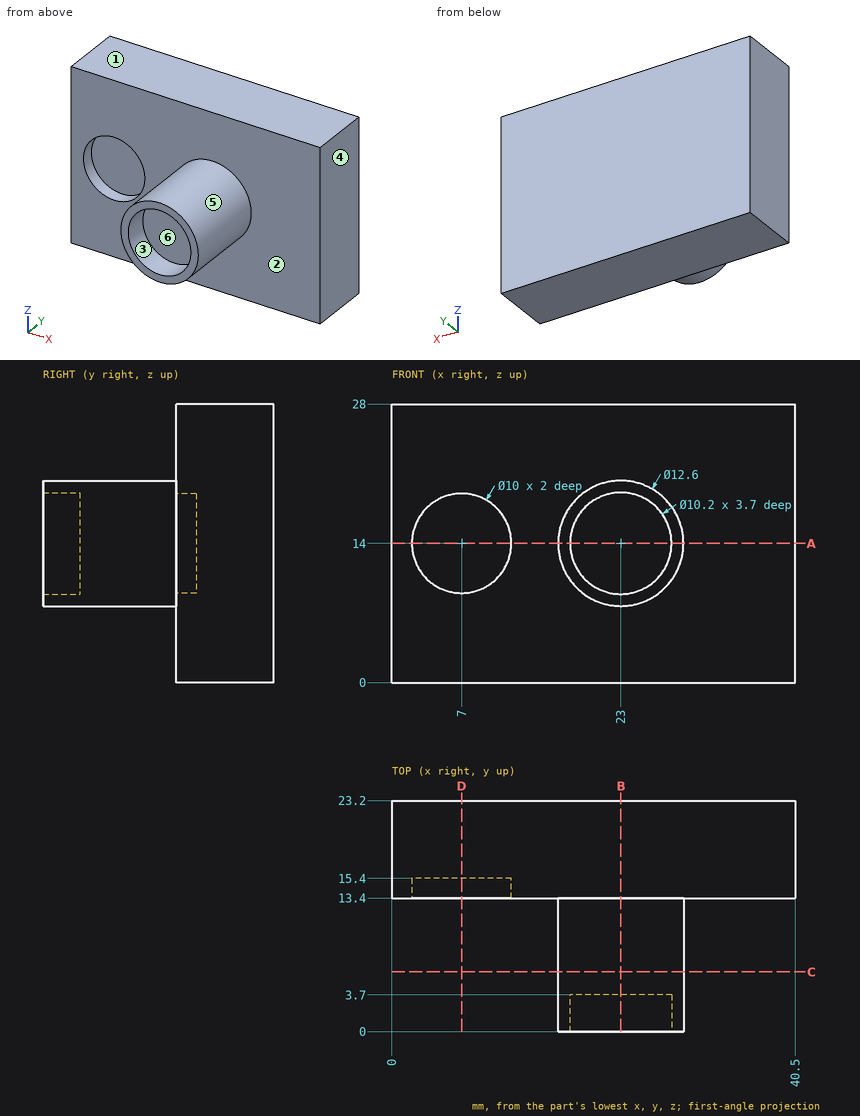
The figure shows three views and two pictorial views of one solid part (mm, origin at its lowest corner). Answer the questions. A direction names the side the tool comes from. Give positions to 0.01 mm unless a question says otherwise; leave off trailing zeros. Write each loop counter-clockwise with the first axis right and the second up, starting at its lowest first coordinate (ties: lowest second). Pieces come first, ordered by that corner, then holes. Notation, with made-up numbers: (-26, 11.5) -> (33, 11.5) arc R25 cw to (33, 38.5) -> close; hole circle Ø6 at (-27.75, 51.5). An arc over 180 degrees is marked (long way). Answer as a JSON object with one key per item and string values.
1) Straight lines are drawn through the part: probe 1 along Z at (x, y) = (7, 13.9); probe 2 along Z at (x, y) = (23, 2.1); probe 3 along Y at (x, z) = (34.5, 16.25). For each, find the intervals that lie inside material, in ascending order. Write a range as from..to.
Findings below:
{"probe 1": "z = 0..9, 19..28", "probe 2": "z = 7.7..8.9, 19.1..20.3", "probe 3": "y = 13.4..23.2"}
2) Flat-ended cylindrical pins translate along their axes: pin 1 Ø5 at (x, z) = (21, 12.5) entering from -Y; pin 2 Ø12 at (y, z) = (12, 23.5) entering from -X; pin 3 Ø8 at (y, z) = (5, 6) entering from -X; pin 4 Ø8 at (x, z) = (7, 14) entering from -Y. Find the tip coordinate at first contact, or state that the pin passes through.
Findings below:
{"pin 1": "stops at y = 3.7", "pin 2": "stops at x = 0", "pin 3": "stops at x = 18.13", "pin 4": "stops at y = 15.4"}
3) Section A-A on z = 14 is taken. Write down the section's boundary in (x, y), then the cut area to 3 significant figures.
Findings below:
{"outline": "(0, 13.4) -> (2, 13.4) -> (2, 15.4) -> (12, 15.4) -> (12, 13.4) -> (16.7, 13.4) -> (16.7, 0) -> (17.9, 0) -> (17.9, 3.7) -> (28.1, 3.7) -> (28.1, 0) -> (29.3, 0) -> (29.3, 13.4) -> (40.5, 13.4) -> (40.5, 23.2) -> (0, 23.2) -> close", "area": "508 mm^2"}
4) Section B-B on x = 23 is taken. Write down the section's boundary in (y, z).
Findings below:
{"outline": "(0, 7.7) -> (13.4, 7.7) -> (13.4, 0) -> (23.2, 0) -> (23.2, 28) -> (13.4, 28) -> (13.4, 20.3) -> (0, 20.3) -> (0, 19.1) -> (3.7, 19.1) -> (3.7, 8.9) -> (0, 8.9) -> close"}
5) For a pull along X with two mould halves and no side action, classify the marked faces 3, 4, 5 and 6 as pulls with the +X half, pulls with the -X half, needs draft (parallel to the pull), parting line crosses it, or undercut.
Findings below:
{"face 3": "undercut", "face 4": "pulls with the +X half", "face 5": "parting line crosses it", "face 6": "undercut"}
6) A tool of negligible diameter and unlimited length cuts with its end or side. For the marked faces 1 and 2, from which of +Z, -Z, +X, -X, +Y, -Y can it reach the whole face along a straight path? Write none if from no direction.
Findings below:
{"face 1": "+Z, +X, -X, +Y, -Y", "face 2": "-Y"}
7) Section D-D on x = 7 is taken. Write down the section's boundary in (y, z), then the cut area to 3 significant figures.
Findings below:
{"outline": "(13.4, 0) -> (23.2, 0) -> (23.2, 28) -> (13.4, 28) -> (13.4, 19) -> (15.4, 19) -> (15.4, 9) -> (13.4, 9) -> close", "area": "254 mm^2"}
8) Section C-C on y = 6 is taken. Write down the section's boundary in (x, z), then the cut area to 3 significant figures.
Findings below:
{"outline": "circle Ø12.6 at (23, 14)", "area": "125 mm^2"}
